Design review of the part built by this model. Coordinates are the model's own, in mm. A direction names the side the tool comes from. Give positions to 0.01 mm unless a question says otherwise; leave off trailing zeros. Loops run counter-clockwise (first coordinate to the right, second up) from the corner with the lowest first, then second, coordinate; pieces in that order, holes last. Notation, with made-up numbers: M 79.25,59 L 108.25,59 A13 ccw 108.25,73 Z; hole C 1,34 d1. An arc over 180 degrees is marked long. Use a Markdown table: item, result. Add a question column.
(1) Add section C-C, the plane z = 9.75. Give the boundary of the cut face in (x, y), then the cut area to 3 significant figures.
(2) Add section A-A, the plane x = -3.75. Give the boundary of the cut face in (y, z), then the cut area to 3 significant figures.
(3) Add section B-B, the plane z = 1.25. Give the boundary of the cut face in (x, y).
(4) Draft analysis for pull direction X (two halves, no side actions). For faces 6 (the face through (-6.213, 0, 2)), 7 (the face through (4, -2.114, 8)), 8 (the face through (5, 1, 2)), state which applies: pulls with the +X half, pulls with the -X half, needs draft (parallel to the pull), parting line crosses it, or undercut.
(5) For probe 1 along X at (y, z) = (0.25, 0.75); probe 2 along X at (y, z) = (-4.5, 5.25); probe 3 along Z at (x, y) = (2.25, -0.25), list the stretches that pass through material, from the lowest coordinate up.
(6) Insertion check: pin 1 Ø0.8 at (y, z) = (-5, 4.5) entering from +X; pin 2 Ø1.5 at (x, y) = (5, 0.5) entering from +Z; pin 3 Ø1.2 at (x, y) = (-4.21, 0.39) entering from +Z; pin 4 Ø1.6 at (y, z) = (-2.5, 5.5) entering from +X. Each pin has a flat end and moves straight along its axis. Give the tip position at first contact, or say it passes through.
(7) Add section D-D, the plane y = 2.5. Give the boundary of the cut face in (x, z).
(8) For faces 1 (the face through (1.787, -4.6, 5.4)), 2 (the face through (-3, 2.886, 2)), 3 (the face through (-3, -2.114, 2)), 4 (the face through (4, 0, 4)), 5 (the face through (4, 2.886, 2)), list the 3-axis set-ups (+Z, -Z, +X, -X, +Y, -Y) from which the entire face can be reached by the end or side of a thin tool; tool diameter is ignored.
Autodesk Inventor part; units mm, degrees
ref_plane "YZ Plane" through (0, 0, 0) normal (1, 0, 0) x (0, 1, 0)
ref_plane "XZ Plane" through (0, 0, 0) normal (0, 1, 0) x (-1, 0, 0)
ref_plane "XY Plane" through (0, 0, 0) normal (0, 0, 1) x (1, 0, 0)
sketch "Sketch1" plane through (0, 0, 0) normal (0, 0, 1) x (1, 0, 0)
  line L0 (-6.2132, 2.886) -> (8.7868, 2.886)
  line L1 (8.7868, 2.886) -> (8.7868, -2.114)
  line L2 (8.7868, -2.114) -> (-6.2132, -2.114)
  line L3 (-6.2132, -2.114) -> (-6.2132, 2.886)
  point P0 (0, 0)
  dimension "d0" = 15
  dimension "d1" = 5
extrude "Extrusion1" add sketch "Sketch1" along normal blind 4
sketch "Sketch2" plane through (0, 0, 0) normal (0, 0, -1) x (-1, 0, 0)
  line L0 (-8.7868, 2.886) -> (6.2132, 2.886)
  line L1 (6.2132, 2.886) -> (6.2132, -2.114)
  point P0 (0, 0)
  point P1 (4.2132, 0.386)
  point P2 (-5.7868, 0.386)
  dimension "d4" = 2.5
  dimension "d5" = 2.5
  dimension "d6" = 2
  dimension "d7" = 10
hole "Hole1" at (-4.2132, 0.386, 0) at (5.7868, 0.386, 0) direction (0, 0, 1) diameter 2 depth 4 tip angle 118
sketch "Sketch3" plane through (0, 0, 0) normal (0, 0, -1) x (-1, 0, 0)
  line L0 (-8.7868, 2.886) -> (6.2132, 2.886)
  line L1 (0.2132, 2.886) -> (-1.7868, 2.886)
  line L2 (-1.7868, 2.886) -> (-1.7868, -7.114)
  line L3 (-1.7868, -7.114) -> (0.2132, -7.114)
  line L4 (0.2132, -7.114) -> (0.2132, 2.886)
  line L5 (6.2132, 2.886) -> (6.2132, -2.114)
  line L6 (-1.7868, 2.886) -> (0.2132, 2.886)
  line L7 (0.2132, 2.886) -> (0.2132, 4.886)
  line L8 (0.2132, 4.886) -> (-1.7868, 4.886)
  line L9 (-1.7868, 4.886) -> (-1.7868, 2.886)
  point P0 (0, 0)
  dimension "d15" = 6
  dimension "d16" = 2
  dimension "d17" = 12
  dimension "d18" = 2
extrude "Extrusion2" add sketch "Sketch3" against normal blind 11
fillet "Fillet1" radius 2 2 edges at (8.7868, 2.886, 2) (8.7868, -2.114, 2)
sketch "Sketch4" plane through (1.7868, -2.114, 0) normal (0, -1, 0) x (1, 0, 0)
  line L0 (0, 0) -> (0, 11)
  line L1 (7, 0) -> (5, 0)
  line L2 (0, 11) -> (5, 11)
  line L3 (5, 11) -> (5, 0)
  line L4 (5, 0) -> (0, 0)
  line L5 (0, 0) -> (0, 11)
  point P0 (-1.7868, 0)
extrude "Extrusion3" add sketch "Sketch4" along normal blind 2
sketch "Sketch5" plane through (-0.2132, -7.114, 0) normal (0, -1, 0) x (1, 0, 0)
  line L0 (-6, 0) -> (-6, 4)
  line L1 (7, 11) -> (2, 11)
  line L2 (-6, 0) -> (7, 0)
  line L3 (7, 0) -> (7, 11)
  line L4 (7, 11) -> (-6, 11)
  line L5 (-6, 11) -> (-6, 0)
  point P0 (0.2132, 0)
  point P1 (2, 11)
extrude "Extrusion4" cut sketch "Sketch5" against normal blind 2
properties part number "oled_support"
Established:
| question | item | result |
|---|---|---|
| 1 | outline | M -0.21,-5.11 L 1.79,-5.11 L 1.79,-4.11 L 6.79,-4.11 L 6.79,-2.11 L 1.79,-2.11 L 1.79,4.89 L -0.21,4.89 Z |
| 1 | area | 30.0 mm^2 |
| 2 | outline | M -2.11,0 L -0.5,0 L -0.5,4 L -2.11,4 Z; M 1.27,0 L 2.89,0 L 2.89,4 L 1.27,4 Z |
| 2 | area | 12.9 mm^2 |
| 3 | outline | M -6.21,-2.11 L -0.21,-2.11 L -0.21,-5.11 L 1.79,-5.11 L 1.79,-4.11 L 6.79,-4.11 L 6.79,-2.11 A2 ccw 8.79,-0.11 L 8.79,0.89 A2 ccw 6.79,2.89 L 1.79,2.89 L 1.79,4.89 L -0.21,4.89 L -0.21,2.89 L -6.21,2.89 Z; hole C -4.21,0.39 d2; hole C 5.79,0.39 d2 |
| 4 | face 6 | pulls with the -X half |
| 4 | face 7 | needs draft |
| 4 | face 8 | undercut |
| 5 | probe 1 | -6.21 to -5.2, -3.22 to 4.8, 6.78 to 8.79 |
| 5 | probe 2 | -0.21 to 1.79 |
| 5 | probe 3 | 0 to 4 |
| 6 | pin 1 | x = 1.79 |
| 6 | pin 2 | z = 4 |
| 6 | pin 3 | through |
| 6 | pin 4 | x = 6.79 |
| 7 | outline | M -6.21,0 L 7.97,0 L 7.97,4 L 1.79,4 L 1.79,11 L -0.21,11 L -0.21,4 L -6.21,4 Z |
| 8 | face 1 | +Z, -Z, +X, -Y |
| 8 | face 2 | +Z, -Z, -X, +Y |
| 8 | face 3 | +Z, -Z, -X, -Y |
| 8 | face 4 | +Z, +X, +Y |
| 8 | face 5 | +Z, -Z, +X, +Y |
